from build123d import *

# Parameters (mm, degrees)
F1_DEPTH = 107.5
F2_W     = 21.5
F2_H     = 6
F2_R     = 12
F3_DEPTH = 25
F4_R     = 7.25
F5_DEPTH = 5


with BuildPart() as f1:
    # F0 (on Front) → F1 (new body, symmetric)
    with BuildSketch(Plane.XZ):
        with BuildLine():
            Line((-6.4, 0), (0, 0))
            Line((0, 0), (6.4, 0))
            ThreePointArc((6.4, 0), (8.662742, 0.937258), (9.6, 3.2))
            Line((9.6, 3.2), (9.6, 42.6))
            Line((9.6, 42.6), (8, 42.6))
            Line((8, 42.6), (8, 3.2))
            ThreePointArc((8, 3.2), (7.531371, 2.068629), (6.4, 1.6))
            Line((6.4, 1.6), (0, 1.6))
            Line((0, 1.6), (-6.4, 1.6))
            ThreePointArc((-6.4, 1.6), (-7.531371, 2.068629), (-8, 3.2))
            Line((-8, 3.2), (-8, 42.6))
            Line((-8, 42.6), (-9.6, 42.6))
            Line((-9.6, 42.6), (-9.6, 3.2))
            ThreePointArc((-9.6, 3.2), (-8.662742, 0.937258), (-6.4, 0))
        make_face()
    extrude(amount=F1_DEPTH, both=True)

    # F2 (on face) → F3 (cut)
    with BuildSketch(Plane(origin=(-9.6, 0, 0), x_dir=(0, -1, 0), z_dir=(-1, 0, 0))):
        with Locations((-96.75, 39.6)):
            Rectangle(F2_W, F2_H)
        Polygon((-42.5, 0), (-107.5, 20), (-107.5, 0), align=None)
        Polygon((42.5, 0), (107.5, 0), (107.5, 20), align=None)
        with Locations((96.75, 39.6)):
            Rectangle(F2_W, F2_H)
        with Locations((0, 20.5)):
            Circle(F2_R)
    extrude(amount=-F3_DEPTH, mode=Mode.SUBTRACT)

    # F4 (on face) → F5 (cut)
    with BuildSketch(Plane(origin=(0, 0, 0), x_dir=(1, 0, 0), z_dir=(0, 0, -1))):
        with Locations((0, -45)):
            Circle(F4_R)
        with Locations((0, 45)):
            Circle(F4_R)
    extrude(amount=-F5_DEPTH, mode=Mode.SUBTRACT)


solid = f1.part
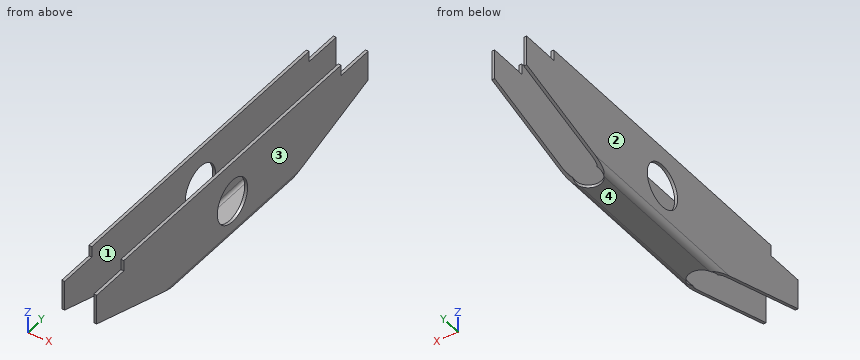
Can you work these out from the model? Positions are in its coordinate system, mm. Face numbers are marked on the shaded views. Round coordinates to 2 decimals unless told otherwise and drop trailing zeros. Write each loop counter-clockwise with the first axis right and the second up, starting at its lowest first coordinate (ties: lowest second). Pieces come first, ordered by that corner, then holes. Notation, with made-up numbers: (44.5, 64.5) -> (93.5, 64.5) arc R15 ccw to (93.5, 68.5) -> close; hole circle Ø7 at (23.25, 44.25). An arc over 180 degrees is marked (long way). Use one line per item in the form item = value. Start each with the question number.
Q1. Imagine slicing it at A-A (y = 0). Please give me the cut outline in (x, z).
Q2. Imagine slicing it at D-D (z = 14). Please give me the cut outline in (x, y).
Q3. I'm going to push flat-ended pins straight in: P1, Ø10, axis at x = 0.5, y = 0, coming from the +Z side; P2, Ø0.5, axis at x = 8.5, z = 40.5, coming from the -Y side; P3, Ø6, axis at x = -3, z = 36.5, coming from the -Y side; P4, Ø1.8, axis at x = -9, y = 95, coming from the +Z side. Where does each tip first touch, or does it pass through?
Q4. Imagine slicing it at C-C (y = -32). Please give me the cut outline in (x, z), then the cut area to 3 significant figures.
Q5. We'd pull the mould along X, two halves only. Please class the marked faces 1, 2, 3 and 4: +X half, -X half, draft (parallel to the pull), parting line (faces both ways), or undercut.
Q6. Imagine slicing it at B-B (z = 6). Please give me the cut outline in (x, y).
Q7. If I drill on probe 1 along X at (y, z) = (-17.5, 16.5); probe 2 along Z at (x, y) = (8.25, 70); probe 3 along Y at (x, z) = (0, 1.2), over which ranges is the centre line in solid material (lowest first)? Write a range as [from, to].
Worked out:
q1.outline = (-9.6, 3.2) arc R3.2 ccw to (-6.4, 0) -> (6.4, 0) arc R3.2 ccw to (9.6, 3.2) -> (9.6, 8.5) -> (8, 8.5) -> (8, 3.2) arc R1.6 cw to (6.4, 1.6) -> (-6.4, 1.6) arc R1.6 cw to (-8, 3.2) -> (-8, 8.5) -> (-9.6, 8.5) -> close; (-9.6, 32.5) -> (-8, 32.5) -> (-8, 42.6) -> (-9.6, 42.6) -> close; (8, 32.5) -> (9.6, 32.5) -> (9.6, 42.6) -> (8, 42.6) -> close
q2.outline = (-9.6, -88) -> (-8, -88) -> (-8, -10.09) -> (-9.6, -10.09) -> close; (-9.6, 10.09) -> (-8, 10.09) -> (-8, 88) -> (-9.6, 88) -> close; (8, -88) -> (9.6, -88) -> (9.6, -10.09) -> (8, -10.09) -> close; (8, 10.09) -> (9.6, 10.09) -> (9.6, 88) -> (8, 88) -> close
q3.P1 = 1.6
q3.P2 = -86
q3.P3 = through
q3.P4 = 36.6
q4.outline = (-9.6, 3.2) arc R3.2 ccw to (-6.4, 0) -> (6.4, 0) arc R3.2 ccw to (9.6, 3.2) -> (9.6, 42.6) -> (8, 42.6) -> (8, 3.2) arc R1.6 cw to (6.4, 1.6) -> (-6.4, 1.6) arc R1.6 cw to (-8, 3.2) -> (-8, 42.6) -> (-9.6, 42.6) -> close
q4.area = 159 mm^2
q5.face_1 = undercut
q5.face_2 = -X half
q5.face_3 = +X half
q5.face_4 = draft
q6.outline = (-9.6, -62) -> (-8, -62) -> (-8, 62) -> (-9.6, 62) -> close; (8, -62) -> (9.6, -62) -> (9.6, 62) -> (8, 62) -> close
q7.probe_1 = [-9.6, -8], [8, 9.6]
q7.probe_2 = [8.46, 42.6]
q7.probe_3 = [-37.75, 37.75]
